Design review of the part built by this model. Coordinates are the model's own, in mm. A direction names the side the tool comes from. Round coordinates to 2 decimals unless told otherwise and drop trailing zeros. Loops run counter-clockwise (first coordinate to the right, second up) from the corner with the lowest first, then second, coordinate; pieces in that order, holes last. Notation, with made-up numbers: M 8.25,-25 L 52.25,-25 A21 ccw 52.25,4 Z; hole C -34,-30.5 d9. An arc over 180 degrees is marked long. One line per item, written item: value. Start each with the question number.
Item 1: Clearance check with flat-ended pins moving along their axes: pin 1 (2 mm diameter, centred on x = 30.5, y = 9.5, fed in from +Z); pin 2 (2.5 mm diameter, centred on y = 9, z = -10, fed in from +X); pin 3 (8 mm diameter, centred on x = 24.5, z = 40.5, fed in from +Y). State where each tip first meets the part, or that it passes through.
Item 2: For line 1 along X through (y, z) = (1.65, 0); line 2 along X through (y, z) = (10.25, 29); line 3 along Y through (x, z) = (-31, 10), list the stretches that pass through material, from the lowest coordinate up.
Item 3: We need section B-B (y = 5.5). Write out the cut boundary in (x, z).
Item 4: We need section A-A (z = -14). Write out the cut boundary in (x, y), then the cut area to 3 significant figures.
Item 5: Mouldability with a two-part tool opening along Z and no side actions: class faces 1 (the flat face through (31, 14, 6)), 2 (the cylindrical face through (-13.55, 2.03, 1.43)), 3 (the flat face through (-31, 9, 30)) as released by +Z, released by -Z, zero draft, split by the parting line, or undercut.
Item 6: We need section C-C (z = 0). Write out the cut boundary in (x, y), then the cut area to 3 significant figures.
Item 7: For faces 4 (the cylindrical face through (-30.972, 10.352, 21.474)), 5 (the flat face through (-29, 9, 6)), 6 (the flat face through (31, 9, 30)), list the 3-axis set-ups (+Z, -Z, +X, -X, +Y, -Y) from which the entire face can be reached by the end or side of a thin tool; tool diameter is ignored.
Item 8: We need section D-D (z = 65). Write out the cut boundary in (x, y).
from build123d import *

# Parameters (mm, degrees)
EXTRUDE_1_DEPTH     = 30
CUT_EXTRUDE_1_REACH = 75.838
SKETCH_2_R          = 2
SKETCH_3_R          = 11
SKETCH_3_R_2        = 1.5
CUT_EXTRUDE_2_DEPTH = 4
SKETCH_4_R          = 13
EXTRUDE_2_DEPTH     = 4
CUT_EXTRUDE_3_REACH = 125.13
SKETCH_5_W          = 12
SKETCH_5_H          = 14


with BuildPart() as part:
    # 草图1 → 凸台-拉伸1 (new, symmetric)
    with BuildSketch(Plane.XY):
        Polygon((33, 0), (-33, 0), (-33, 14), (-29, 14), (-29, 4), (29, 4), (29, 14), (33, 14), align=None)
    extrude(amount=EXTRUDE_1_DEPTH, both=True)

    # 切除-拉伸1: up to this face of the body (flat: up to its plane)
    cut_extrude_1_end = Plane(part.part.faces().sort_by_distance((-33, 7, 0))[0])
    # 草图2 → 切除-拉伸1 (cut, up to the picked face)
    with BuildSketch(Plane(origin=(33, 0, 0), x_dir=(0, 0, -1), z_dir=(1, 0, 0)), mode=Mode.PRIVATE) as cut_extrude_1_sk1:
        with Locations((-20, 9)):
            Circle(SKETCH_2_R)
    cut_extrude_1_tool1 = split(extrude(cut_extrude_1_sk1.sketch, amount=-CUT_EXTRUDE_1_REACH, mode=Mode.PRIVATE), bisect_by=cut_extrude_1_end, keep=Keep.BOTH, mode=Mode.PRIVATE)
    # 草图2 → 切除-拉伸1 (cut, up to the picked face)
    with BuildSketch(Plane(origin=(33, 0, 0), x_dir=(0, 0, -1), z_dir=(1, 0, 0)), mode=Mode.PRIVATE) as cut_extrude_1_sk2:
        with Locations((-10, 9)):
            Circle(SKETCH_2_R)
    cut_extrude_1_tool2 = split(extrude(cut_extrude_1_sk2.sketch, amount=-CUT_EXTRUDE_1_REACH, mode=Mode.PRIVATE), bisect_by=cut_extrude_1_end, keep=Keep.BOTH, mode=Mode.PRIVATE)
    # 草图2 → 切除-拉伸1 (cut, up to the picked face)
    with BuildSketch(Plane(origin=(33, 0, 0), x_dir=(0, 0, -1), z_dir=(1, 0, 0)), mode=Mode.PRIVATE) as cut_extrude_1_sk3:
        with Locations(Location((10, 9, 0), (0, 0, 90))):
            Circle(SKETCH_2_R)
    cut_extrude_1_tool3 = split(extrude(cut_extrude_1_sk3.sketch, amount=-CUT_EXTRUDE_1_REACH, mode=Mode.PRIVATE), bisect_by=cut_extrude_1_end, keep=Keep.BOTH, mode=Mode.PRIVATE)
    # 草图2 → 切除-拉伸1 (cut, up to the picked face)
    with BuildSketch(Plane(origin=(33, 0, 0), x_dir=(0, 0, -1), z_dir=(1, 0, 0)), mode=Mode.PRIVATE) as cut_extrude_1_sk4:
        with Locations((0, 9)):
            Circle(SKETCH_2_R)
    cut_extrude_1_tool4 = split(extrude(cut_extrude_1_sk4.sketch, amount=-CUT_EXTRUDE_1_REACH, mode=Mode.PRIVATE), bisect_by=cut_extrude_1_end, keep=Keep.BOTH, mode=Mode.PRIVATE)
    add(cut_extrude_1_tool1.solids().sort_by(Axis((33, 9, 20), (-1, 0, 0)))[0], mode=Mode.SUBTRACT)
    add(cut_extrude_1_tool2.solids().sort_by(Axis((33, 9, 10), (-1, 0, 0)))[0], mode=Mode.SUBTRACT)
    add(cut_extrude_1_tool3.solids().sort_by(Axis((33, 9, -10), (-1, 0, 0)))[0], mode=Mode.SUBTRACT)
    add(cut_extrude_1_tool4.solids().sort_by(Axis((33, 9, 0), (-1, 0, 0)))[0], mode=Mode.SUBTRACT)

    # 草图3 → 切除-拉伸2 (cut)
    with BuildSketch(Plane(origin=(0, 4, 0), x_dir=(1, 0, 0), z_dir=(0, 1, 0))):
        with Locations(Location((0, 0, 0), (0, 0, 270))):
            Circle(SKETCH_3_R)
        with Locations(Location((0, 14, 0), (0, 0, 270))):
            Circle(SKETCH_3_R_2)
        with Locations(Location((14, 0, 0), (0, 0, 270))):
            Circle(SKETCH_3_R_2)
        with Locations(Location((0, -14, 0), (0, 0, 270))):
            Circle(SKETCH_3_R_2)
        with Locations(Location((-14, 0, 0), (0, 0, 270))):
            Circle(SKETCH_3_R_2)
    extrude(amount=-CUT_EXTRUDE_2_DEPTH, mode=Mode.SUBTRACT)

    # 草图4 → 凸台-拉伸2 (add)
    with BuildSketch(Plane.XZ):
        with BuildLine():
            Line((-33, 30), (33, 30))
            Line((33, 30), (33, 70))
            ThreePointArc((33, 70), (0, 103), (-33, 70))
            Line((-33, 70), (-33, 30))
        make_face()
        with Locations(Location((0, 70, 0), (0, 0, 270))):
            Circle(SKETCH_4_R, mode=Mode.SUBTRACT)
    extrude(amount=-EXTRUDE_2_DEPTH)

    # 切除-拉伸3: up to this face of the body (flat: up to its plane)
    cut_extrude_3_end = Plane(part.part.faces().sort_by_distance((-33, 6.051807691, 8.158777474))[0])
    # 草图5 → 切除-拉伸3 (cut, up to the picked face)
    with BuildSketch(Plane(origin=(33, 0, 0), x_dir=(0, 0, -1), z_dir=(1, 0, 0)), mode=Mode.PRIVATE) as cut_extrude_3_sk1:
        with Locations((24, 7)):
            Rectangle(SKETCH_5_W, SKETCH_5_H)
    cut_extrude_3_tool1 = split(extrude(cut_extrude_3_sk1.sketch, amount=-CUT_EXTRUDE_3_REACH, mode=Mode.PRIVATE), bisect_by=cut_extrude_3_end, keep=Keep.BOTH, mode=Mode.PRIVATE)
    add(cut_extrude_3_tool1.solids().sort_by(Axis((33, 7, -24), (-1, 0, 0)))[0], mode=Mode.SUBTRACT)


solid = part.part
A:
1. pin 1: z = 30
1. pin 2: through
1. pin 3: y = 4
2. line 1: -33 to -15.5, -12.5 to -11, 11 to 12.5, 15.5 to 33
2. line 2: -33 to -29, 29 to 33
2. line 3: 0 to 7, 11 to 14
3. outline: M -33,-18 L -29,-18 L -29,30 L -33,30 Z; M 29,-18 L 33,-18 L 33,30 L 29,30 Z
4. outline: M -33,0 L -1.5,0 L -1.5,4 L -29,4 L -29,14 L -33,14 Z; M 1.5,0 L 33,0 L 33,14 L 29,14 L 29,4 L 1.5,4 Z
4. area: 332 mm2
5. face 1: zero draft
5. face 2: undercut
5. face 3: released by +Z
6. outline: M -33,0 L -15.5,0 L -15.5,4 L -29,4 L -29,7 L -33,7 Z; M -33,11 L -29,11 L -29,14 L -33,14 Z; M -12.5,0 L -11,0 L -11,4 L -12.5,4 Z; M 11,0 L 12.5,0 L 12.5,4 L 11,4 Z; M 15.5,0 L 33,0 L 33,7 L 29,7 L 29,4 L 15.5,4 Z; M 29,11 L 33,11 L 33,14 L 29,14 Z
6. area: 200 mm2
7. face 4: +X, -X
7. face 5: +Z, -Z, +Y
7. face 6: +Z, +X, -X, +Y
8. outline: M -33,0 L -12,0 L -12,4 L -33,4 Z; M 12,0 L 33,0 L 33,4 L 12,4 Z
